from build123d import *

# Parameters (mm, degrees)
SKETCH_1_W      = 17.78
SKETCH_1_H      = 12.7
SKETCH_1_R      = 1
SKETCH_1_W_2    = 2.9
SKETCH_1_H_2    = 4.9
EXTRUDE_1_DEPTH = 1
SKETCH_1_3_W    = 2.9
SKETCH_1_3_H    = 4.9
EXTRUDE_2_DEPTH = 2.1


with BuildPart() as part:
    # 草图1 → 凸台-拉伸1 (new body)
    # profile 1 of 2: a face of its own
    with BuildSketch(Plane(origin=(0, 0, 0), x_dir=(1, 0, 0), z_dir=(0, 1, 0))):
        Rectangle(SKETCH_1_W, SKETCH_1_H)
        with Locations(Location((6.35, 3.9, 0), (0, 0, 270))):
            Circle(SKETCH_1_R, mode=Mode.SUBTRACT)
        with Locations(Location((-6.35, 3.9, 0), (0, 0, 270))):
            Circle(SKETCH_1_R, mode=Mode.SUBTRACT)
        with Locations((0, 0.9)):
            Rectangle(SKETCH_1_W_2, SKETCH_1_H_2, mode=Mode.SUBTRACT)
    # profile 2 of 2: a face of its own
    with BuildSketch(Plane(origin=(0, 0, 0), x_dir=(1, 0, 0), z_dir=(0, 1, 0))):
        with Locations((0, 0.9)):
            Rectangle(SKETCH_1_W_2, SKETCH_1_H_2)
    extrude(amount=EXTRUDE_1_DEPTH)

    # 草图1<3> → 凸台-拉伸2 (add)
    with BuildSketch(Plane(origin=(0, 0, 0), x_dir=(1, 0, 0), z_dir=(0, 1, 0))):
        with Locations((0, 0.9)):
            Rectangle(SKETCH_1_3_W, SKETCH_1_3_H)
    extrude(amount=EXTRUDE_2_DEPTH)


solid = part.part
Could you check a few things on this model? Use its own coordinates, in mm. A direction names the side the tool comes from. Give positions to 0.01 mm unless a question says otherwise; leave off trailing zeros. Order: outer loops, then holes, each group sorted by start corner. A loop starts at its lowest first (then second) coordinate and runs counter-clockwise, first axis right, second up. Notation, with made-up numbers: (78.25, 79) -> (134.25, 79) arc R27 cw to (134.25, 110) -> close; hole circle Ø11 at (-20.75, 64). An arc over 180 degrees is marked (long way). Return JSON: item names as keys, results as strings.
1. Imagine slicing it at A-A on z = -3.9. List the corners of the cut face in (x, y) for me, then the cut area to 3 significant figures.
Answer list:
{"outline": "(-8.89, 0) -> (-7.35, 0) -> (-7.35, 1) -> (-8.89, 1) -> close; (-5.35, 0) -> (5.35, 0) -> (5.35, 1) -> (-5.35, 1) -> close; (7.35, 0) -> (8.89, 0) -> (8.89, 1) -> (7.35, 1) -> close", "area": "13.8 mm2"}
2. Imagine slicing it at D-D on z = -1. List the corners of the cut face in (x, y) for me, then the cut area to 3 significant figures.
Answer list:
{"outline": "(-8.89, 0) -> (8.89, 0) -> (8.89, 1) -> (1.45, 1) -> (1.45, 2.1) -> (-1.45, 2.1) -> (-1.45, 1) -> (-8.89, 1) -> close", "area": "21.0 mm2"}
3. I need wall thicknesses on line 1 (X direction, y = 0.4, z = -3.9); line 2 (X direction, y = 0.2, z = -4.5); line 3 (Y direction, x = 3, z = 5.5). Which ranges of each line are inside material? Lowest first, please. Write a range as from..to.
Answer list:
{"line 1": "x = -8.89..-7.35, -5.35..5.35, 7.35..8.89", "line 2": "x = -8.89..-7.15, -5.55..5.55, 7.15..8.89", "line 3": "y = 0..1"}
4. For pin 1 Ø3 at (x, z) = (6.5, 1.5) entering from +Y; pin 2 Ø2.5 at (x, z) = (-6.35, -3.9) entering from -Y; pin 3 Ø0.6 at (y, z) = (1.5, -0.5) entering from +X; pin 4 Ø0.9 at (x, y) = (0, 1.5) entering from +Z, each with a flat end and sliding along its axis, tell me the tip position at first contact or that it passes through.
Answer list:
{"pin 1": "stops at y = 1", "pin 2": "stops at y = 0", "pin 3": "stops at x = 1.45", "pin 4": "stops at z = 1.55"}
5. Imagine slicing it at C-C on y = 0.5. List the corners of the cut face in (x, z) for me.
Answer list:
{"outline": "(-8.89, -6.35) -> (8.89, -6.35) -> (8.89, 6.35) -> (-8.89, 6.35) -> close; hole circle Ø2 at (-6.35, -3.9); hole circle Ø2 at (6.35, -3.9)"}
6. Imagine slicing it at B-B on x = -6.35. List the corners of the cut face in (y, z) for me, then the cut area to 3 significant figures.
Answer list:
{"outline": "(0, -6.35) -> (1, -6.35) -> (1, -4.9) -> (0, -4.9) -> close; (0, -2.9) -> (1, -2.9) -> (1, 6.35) -> (0, 6.35) -> close", "area": "10.7 mm2"}
7. On a 3-axis mill with a long thin cutter (end or side, diameter ignored), from which of +Z, -Z, +X, -X, +Y, -Y can I reach the whole of each face in a straight line? I mean faces 1 (the flat face through (0, 1.5, 1.55)), 2 (the flat face through (-0.1, 0.5, -6.35)), 3 (the flat face through (-1.45, 1.5, -0.9)), 4 (the flat face through (0, 1.5, -3.35)). Say none if no direction works.
Answer list:
{"face 1": "+Z, +X, -X, +Y", "face 2": "-Z, +X, -X, +Y, -Y", "face 3": "+Z, -Z, -X, +Y", "face 4": "-Z, +X, -X, +Y"}
8. Thinking about a two-plate mould opening in Z: for faces 5 (the cylindrical face through (5.374, 0.493, -4.117)), 6 (the flat face through (-0.1, 0.5, 6.35)), 7 (the flat face through (1.45, 1.5, -0.9)), which applies, pulls with the +Z half, pulls with the -Z half, needs draft (parallel to the pull), parting line crosses it, or undercut?
Answer list:
{"face 5": "undercut", "face 6": "pulls with the +Z half", "face 7": "needs draft"}
